Verification items for the finished model (mm, model axes). A direction names the side the tool comes from. Give positions to 0.01 mm unless a question says otherwise; leave off trailing zeros. Order: outer loops, then holes, each group sorted by start corner. A loop starts at its lowest first (then second) coordinate and runs counter-clockwise, first axis right, second up. Notation, with made-up numbers: (-12.5, 41) -> (21.5, 41) arc R22 cw to (21.5, 47) -> close; hole circle Ø1 at (-20.75, -23). An arc over 180 degrees is marked (long way). Return JSON: item names as keys, results as strings. Group by question number.
(1) Cross-section at B-B on x = -16. Enter the section's corners in (y, z).
(2) Cross-section at C-C on z = 151. Enter the section's corners in (x, y).
(3) Depth check by flat-ended pin: pin 1 Ø3.5 at (y, z) = (49, 301.5) entering from -X; pin 2 Ø4 at (x, z) = (33, 255) entering from +Y; pin 3 Ø3.5 at (x, z) = (48.5, 73.5) entering from -Y. Enter the tip coordinate at first touch or a pass-through.
(4) Cross-section at A-A on y = -35. Enter the section's corners in (x, z).
(5) Release check for a two-part mould opening along X. For faces 1 (the face through (50, 1, 219)), 2 (the face through (1, -47, 220)), 3 (the face through (-47.5, -43.7, 0)) record: pulls with the +X half, pulls with the -X half, needs draft (parallel to the pull), parting line crosses it, or undercut.
(6) Cross-section at D-D on z = 324.5. Enter the section's corners in (x, y), then the cut area to 3 significant figures.
(7) Tool access check on faces 4 (the face through (48, -15, 415)), 5 (the face through (-47, -1, 219)). Record the directions out of +Z, -Z, +X, -X, +Y, -Y that give a thin tool (end or side, any length) a straight path to the whole face; none if there is none.
(8) Thickness scan on line 1 along X through (y, z) = (27.5, 300); line 2 along Y through (x, z) = (31.5, 288). Record the ranges inside material, lowest first.
Autodesk Inventor part; units mm, degrees
ref_plane "Start Plane" through (0, 0, 0) normal (0, 0, 1) x (1, 0, 0)
ref_plane "End Plane" through (0, 0, 450) normal (0, 0, 1) x (1, 0, 0)
ref_plane "Work Plane5" through (0, -50, 450) normal (0, 0.7071, 0.7071) x (1, 0, 0)
ref_plane "Start Plane" through (0, 0, 0) normal (0, 0, 1) x (1, 0, 0)
ref_plane "End Plane" through (0, 0, 450) normal (0, 0, 1) x (1, 0, 0)
sketch "Sketch" plane through (0, 0, 0) normal (0, 0, 1) x (1, 0, 0)
  line L0 (-50, -44) -> (-50, 44)
  line L1 (-44, 50) -> (44, 50)
  line L2 (50, 44) -> (50, -44)
  line L3 (44, -50) -> (-44, -50)
  arc A0 (-50, -44) -> (-44, -50) centre (-44, -44) ccw
  arc A1 (50, 44) -> (44, 50) centre (44, 44) ccw
  arc A2 (-44, 50) -> (-50, 44) centre (-44, 44) ccw
  arc A3 (44, -50) -> (50, -44) centre (44, -44) ccw
  arc A4 (-44, 47) -> (-47, 44) centre (-44, 44) ccw
  line L4 (-44, 47) -> (44, 47)
  arc A5 (47, 44) -> (44, 47) centre (44, 44) ccw
  line L5 (47, 44) -> (47, -44)
  arc A6 (44, -47) -> (47, -44) centre (44, -44) ccw
  line L6 (44, -47) -> (-44, -47)
  arc A7 (-47, -44) -> (-44, -47) centre (-44, -44) ccw
  line L7 (-47, -44) -> (-47, 44)
  line L8 (0, 71.7397) -> (0, -71.7397) construction
  line L9 (-71.7397, 0) -> (71.7397, 0) construction
  dimension "d7" = 6
  dimension "d9" = 100
  dimension "d11" = 100
  dimension "d12" = 3
  dimension "d15" = 50
  dimension "d16" = 50
extrude "Body" add sketch "Sketch" along normal up to surface (450 mm away) from surface at 0
sketch "Sketch3" plane through (0, 0, 0) normal (0, 0, 1) x (1, 0, 0)
  line L0 (0, 0) -> (10, 0)
ref_plane "Work Plane3" through (0, 0, 0) normal (0, -1, 0) x (1, 0, 0)
sketch "Sketch5" plane through (44, 50, 450) normal (0, 1, 0) x (1, 0, 0)
  line L0 (-88, 0) -> (0, 0)
  line L1 (0, 450) -> (0, 0)
  line L2 (-88, 0) -> (0, 0)
  line L3 (0, 0) -> (0, 141.42)
  line L4 (0, 141.42) -> (-88, 141.42)
  line L5 (-88, 141.42) -> (-88, 0)
  point P0 (-44, 450)
  point P1 (-44, 0)
  point P2 (-44, 141.42)
  dimension "d19" = 141.42
extrude "Extrusion2" cut sketch "Sketch5" against normal blind 10
sketch "Sketch6" plane through (0, 0, 0) normal (0, 0, -1) x (-1, 0, 0)
  line L0 (44, 50) -> (-44, 50)
  line L1 (-44, -50) -> (44, -50)
  line L2 (30, 50) -> (28, 50)
  line L3 (28, 50) -> (28, -50)
  line L4 (28, -50) -> (30, -50)
  line L5 (30, -50) -> (30, 50)
  line L6 (50, -44) -> (50, 44)
  line L7 (50, -30) -> (-50.0252, -30)
  line L8 (-50.0252, -30) -> (-50.0252, -28)
  line L9 (-50.0252, -28) -> (50, -28)
  line L10 (50, -28) -> (50, -30)
  line L11 (-28, -50) -> (-30, -50)
  line L12 (-30, -50) -> (-30, 50)
  line L13 (-30, 50) -> (-28, 50)
  line L14 (-28, 50) -> (-28, -50)
  line L15 (-50, 44) -> (-50, -44)
  line L16 (50, 30) -> (-50, 30)
  line L17 (-50, 30) -> (-50, 28)
  line L18 (-50, 28) -> (50, 28)
  line L19 (50, 28) -> (50, 30)
  point P0 (0, 0)
  point P1 (30, -30)
  point P2 (30, -28)
  point P3 (30, 28)
  point P4 (30, 30)
  point P5 (28, 30)
  point P6 (-28, 30)
  point P7 (-30, 30)
  point P8 (-50, 30)
  point P9 (-30, 28)
  point P10 (-30, -28)
  point P11 (-30, -30)
  point P12 (-28, -30)
  point P13 (28, -30)
  point P14 (28, -28)
  point P15 (-28, -28)
  point P16 (-28, 28)
  point P17 (28, 28)
  dimension "d22" = 2
  dimension "d23" = 2
  dimension "d24" = 20
  dimension "d25" = 20
  dimension "d26" = 2
  dimension "d27" = 2
  dimension "d28" = 20
  dimension "d29" = 20
extrude "Extrusion3" cut sketch "Sketch6" against normal blind 100 contours L5 L16 L3 L0 | L16 L6 L18 L5 | L5 L18 L3 L16 | L14 L16 L12 L0 | L3 L18 L14 L16 | L5 L9 L3 L18 | L14 L18 L12 L16 | L9 L6 L7 L5 | L5 L7 L3 L9 | L12 L18 L15 L16 | L14 L9 L12 L18 | L3 L7 L14 L9 | L5 L1 L3 L7 | L14 L7 L12 L9 | L12 L7 L15 L9 | L14 L1 L12 L7 | L15 L7 L8 L9
ref_plane "Work Plane5" through (0, -50, 450) normal (0, 0.7071, 0.7071) x (1, 0, 0)
split "Split2" plane through (0, -50, 450) removes the side toward (0, 0.7071, 0.7071)
sketch "Sketch7" plane through (-44, 50, 308.58) normal (0, 1, 0) x (1, 0, 0)
  line L0 (0, 0) -> (0, -44.42)
  line L1 (88, 308.58) -> (88, -138.42)
  line L2 (0, 0) -> (88, 0)
  line L3 (88, 0) -> (88, 97.42)
  line L4 (88, 97.42) -> (0, 97.42)
  line L5 (0, 97.42) -> (0, 0)
  point P0 (44, 308.58)
  point P1 (88, 0)
  dimension "d32" = 97.42
extrude "Extrusion4" cut sketch "Sketch7" against normal blind 5
sketch "Sketch4" plane through (0, 0, 0) normal (0, -1, 0) x (1, 0, 0)
  line L0 (-2, 0) -> (12, 0)
  line L1 (-2, 450) -> (12, 450)
  dimension "d18" = 450
equation "\"d7\" = G_IR"
equation "\"d9\" = G_W"
equation "\"d11\" = G_H"
equation "\"d12\" = G_T"
equation "\"d15\" = 0.5 * d9"
equation "\"d16\" = 0.5 * d11"
equation "\"d3\" = G_L"
equation "\"d23\" = d22"
equation "\"d26\" = d22"
equation "\"d27\" = d22"
equation "\"G_W\" = 100"
equation "\"G_H\" = 100"
equation "\"G_T\" = 3"
equation "\"G_IR\" = 6"
equation "\"G_L\" = d18"
equation "\"G_OFFSET_START\" = 0"
properties part number "ISO 10799-2 - 100x100x3 - 450" material "Steel, Mild"
Verdict:
{
 "1": {"outline": "(-50, 0) -> (-47, 0) -> (-47, 447) -> (-50, 450) -> close; (47, 0) -> (50, 0) -> (50, 211.16) -> (47, 211.16) -> close"},
 "2": {"outline": "(-50, -44) arc R6 ccw to (-44, -50) -> (44, -50) arc R6 ccw to (50, -44) -> (50, 44) arc R6 ccw to (44, 50) -> (-44, 50) arc R6 ccw to (-50, 44) -> close; hole (-47, -44) arc R3 ccw to (-44, -47) -> (44, -47) arc R3 ccw to (47, -44) -> (47, 44) arc R3 ccw to (44, 47) -> (-44, 47) arc R3 ccw to (-47, 44) -> close"},
 "3": {"pin 1": "x = -49.04", "pin 2": "y = -47", "pin 3": "y = -49.33"},
 "4": {"outline": "(-50, 0) -> (-47, 0) -> (-47, 435) -> (-50, 435) -> close; (47, 0) -> (50, 0) -> (50, 435) -> (47, 435) -> close"},
 "5": {"face 1": "pulls with the +X half", "face 2": "undercut", "face 3": "needs draft"},
 "6": {"outline": "(-50, -44) arc R6 ccw to (-44, -50) -> (44, -50) arc R6 ccw to (50, -44) -> (50, 44) arc R6 ccw to (44, 50) -> (44, 47) arc R3 cw to (47, 44) -> (47, -44) arc R3 cw to (44, -47) -> (-44, -47) arc R3 cw to (-47, -44) -> (-47, 44) arc R3 cw to (-44, 47) -> (-44, 50) arc R6 ccw to (-50, 44) -> close", "area": "877 mm²"},
 "7": {"face 4": "+Z, +X, -X, +Y", "face 5": "+Z, -Z"},
 "8": {"line 1": "-50 to -47, 47 to 50", "line 2": "-50 to -47"}
}
